from build123d import *

# Parameters (mm, degrees)
SKETCH_R             = 1.375
PAD_DEPTH            = 3
FILLET_R             = 3.5
SKETCH001_W          = 95
SKETCH001_H          = 120
SKETCH001_R          = 1.375
SKETCH001_R_2        = 1.4
SKETCH001_R_3        = 1.403567
PAD001_DEPTH         = 7
SKETCH002_R          = 2.75
POCKET_DEPTH         = 1.75
SKETCH003_W          = 65
SKETCH003_H          = 67.5
POCKET001_DEPTH      = 4
SKETCH004_W          = 65
SKETCH004_H          = 100
PAD002_DEPTH         = 5
SKETCH005_W          = 70
SKETCH005_H          = 102.5
PAD003_DEPTH         = 3
SKETCH006_W          = 70
SKETCH006_H          = 5
POCKET002_DEPTH      = 5
FILLET001_R          = 1.5
SKETCH008_R          = 2.54
SKETCH008_R_2        = 1.27
SKETCH008_R_3        = 9.919017
PAD004_DEPTH         = 2
PAD004_FACE95_R      = 2.54
PAD004_FACE95_R_2    = 1.27
PAD005_DEPTH         = 1
PAD005_FACE94_R      = 2.54
PAD005_FACE94_R_2    = 1.27
PAD006_DEPTH         = 1
SKETCH009_W          = 12.7
SKETCH009_H          = 12.7
POCKET003_DEPTH      = 6
POCKET003_DEPTH_BACK = 1
FILLET002_R          = 1.5
SKETCH010_W          = 12.5
SKETCH010_H          = 10
SKETCH010_W_2        = 70
SKETCH010_H_2        = 7.5
PAD007_DEPTH         = 3
SKETCH015_W          = 45
SKETCH015_H          = 35
POCKET004_DEPTH      = 1
SKETCH028_W          = 1.25
SKETCH028_H          = 105
POCKET005_DEPTH      = 5
SKETCH031_W          = 70
SKETCH031_H          = 5
PAD025_DEPTH         = 15
FILLET007_R          = 4.2
SKETCH033_W          = 70
SKETCH033_H          = 7.5
PAD026_DEPTH         = 3.9
BODY_PLACEMENT_ANGLE = 90


with BuildPart() as part:
    # Sketch → Pad (new body)
    with BuildSketch(Plane.XZ):
        Polygon((6.25, 0), (0, 0), (0, 30), (6.25, 30), (58.75, 30), (65, 30), (65, 0), (58.75, 0), (58.75, 11.25), (6.25, 11.25), align=None)
        with Locations((3.5, 26.5)):
            Circle(SKETCH_R, mode=Mode.SUBTRACT)
        with Locations((61.5, 26.5)):
            Circle(SKETCH_R, mode=Mode.SUBTRACT)
        with Locations((3.5, 3.5)):
            Circle(SKETCH_R, mode=Mode.SUBTRACT)
        with Locations((61.5, 3.5)):
            Circle(SKETCH_R, mode=Mode.SUBTRACT)
    extrude(amount=PAD_DEPTH)

    # Fillet
    fillet_edges = [part.edges().sort_by_distance(p)[0] for p in [
        (0, -1.5, 30),
        (0, -1.5, 0),
        (65, -1.5, 30),
        (65, -1.5, 0),
    ]]
    fillet(fillet_edges, radius=FILLET_R)

    # Sketch001 (on Face5 of Fillet) → Pad001 (join)
    with BuildSketch(Plane.XZ.offset(3)):
        with Locations((32.5, 50)):
            Rectangle(SKETCH001_W, SKETCH001_H)
        with Locations((3.5, 26.5)):
            Circle(SKETCH001_R, mode=Mode.SUBTRACT)
        with Locations((3.5, 3.5)):
            Circle(SKETCH001_R_2, mode=Mode.SUBTRACT)
        with Locations((61.5, 3.5)):
            Circle(SKETCH001_R_2, mode=Mode.SUBTRACT)
        with Locations((61.5, 26.5)):
            Circle(SKETCH001_R_3, mode=Mode.SUBTRACT)
    extrude(amount=PAD001_DEPTH)

    # Sketch002 (on Face29 of Pad001) → Pocket (cut)
    with BuildSketch(Plane.XZ.offset(10)):
        with Locations((3.5, 3.499999)):
            Circle(SKETCH002_R)
        with Locations((3.55131, 26.405157)):
            Circle(SKETCH002_R)
        with Locations((61.5, 26.500002)):
            Circle(SKETCH002_R)
        with Locations((61.561516, 3.466109)):
            Circle(SKETCH002_R)
    extrude(amount=-POCKET_DEPTH, mode=Mode.SUBTRACT)

    # Sketch003 (on Face5 of Pocket) → Pocket001 (cut)
    with BuildSketch(Plane(origin=(0, -3, 0), x_dir=(1, 0, 0), z_dir=(0, 1, 0))):
        with Locations((32.5, -66.25)):
            Rectangle(SKETCH003_W, SKETCH003_H)
    extrude(amount=-POCKET001_DEPTH, mode=Mode.SUBTRACT)

    # Sketch004 (on Face5 of Pocket001) → Pad002 (join)
    with BuildSketch(Plane(origin=(0, -3, 0), x_dir=(1, 0, 0), z_dir=(0, 1, 0))):
        Polygon((0, 5), (65, 5), (70, 5), (70, -100), (80, -100), (80, -110), (-15, -110), (-15, -100), (-5, -100), (-5, 5), align=None)
        with Locations((32.5, -50)):
            Rectangle(SKETCH004_W, SKETCH004_H, mode=Mode.SUBTRACT)
    extrude(amount=PAD002_DEPTH)

    # Sketch005 (on Face22 of Pad002) → Pad003 (join)
    with BuildSketch(Plane(origin=(0, 2, 0), x_dir=(1, 0, 0), z_dir=(0, 1, 0))):
        Polygon((75, 5), (-10, 5), (-10, -100), (-15, -100), (-15, -110), (80, -110), (80, -100), (75, -100), align=None)
        with Locations((32.5, -51.25)):
            Rectangle(SKETCH005_W, SKETCH005_H, mode=Mode.SUBTRACT)
    extrude(amount=PAD003_DEPTH)

    # Sketch006 (on Face34 of Pad003) → Pocket002 (cut)
    with BuildSketch(Plane(origin=(0, 5, 0), x_dir=(1, 0, 0), z_dir=(0, 1, 0))):
        with Locations((32.5, 2.5)):
            Rectangle(SKETCH006_W, SKETCH006_H)
    extrude(amount=-POCKET002_DEPTH, mode=Mode.SUBTRACT)

    # Fillet001
    fillet001_edges = [part.edges().sort_by_distance(p)[0] for p in [
        (32.5, -10, -10),
        (-15, -10, 50),
        (80, -10, 50),
        (32.5, -10, 110),
        (58.811516, -10, 3.466109),
        (58.75, -10, 26.500002),
        (0.80131, -10, 26.405157),
        (0.75, -10, 3.499999),
    ]]
    fillet(fillet001_edges, radius=FILLET001_R)

    # Sketch008 (on Face90 of Fillet001) → Pad004 (join)
    with BuildSketch(Plane(origin=(0, -7, 0), x_dir=(1, 0, 0), z_dir=(0, 1, 0))):
        with Locations((43.18, -96.52)):
            Circle(SKETCH008_R)
        with Locations((43.18, -96.52)):
            Circle(SKETCH008_R_2, mode=Mode.SUBTRACT)
        with Locations((60.96, -96.52)):
            Circle(SKETCH008_R)
        with Locations((60.96, -96.52)):
            Circle(SKETCH008_R_2, mode=Mode.SUBTRACT)
        with Locations((52.07, -81.28)):
            Circle(SKETCH008_R_3)
    extrude(amount=PAD004_DEPTH)

    # Pad004 Face95 → Pad005 (add)
    with BuildSketch(Plane(origin=(43.18, -5, 96.52), x_dir=(1, 0, 0), z_dir=(0, 1, 0))):
        Circle(PAD004_FACE95_R)
        Circle(PAD004_FACE95_R_2, mode=Mode.SUBTRACT)
    extrude(amount=PAD005_DEPTH)

    # Pad005 Face94 → Pad006 (add)
    with BuildSketch(Plane(origin=(60.96, -5, 96.52), x_dir=(1, 0, 0), z_dir=(0, 1, 0))):
        Circle(PAD005_FACE94_R)
        Circle(PAD005_FACE94_R_2, mode=Mode.SUBTRACT)
    extrude(amount=PAD006_DEPTH)

    # Sketch009 (on Face57 of Pad006) → Pocket003 (cut, two sides)
    with BuildSketch(Plane(origin=(0, 2, 0), x_dir=(1, 0, 0), z_dir=(0, 1, 0))) as pocket003_sk:
        with Locations((52.07, -105.41)):
            Rectangle(SKETCH009_W, SKETCH009_H)
    extrude(amount=-POCKET003_DEPTH, mode=Mode.SUBTRACT)
    extrude(pocket003_sk.sketch, amount=POCKET003_DEPTH_BACK, mode=Mode.SUBTRACT)

    # Fillet002
    fillet002_edges = [part.edges().sort_by_distance(p)[0] for p in [
        (45.72, -0.5, 110),
        (52.07, -4, 110),
        (58.42, -0.5, 110),
        (52.07, 3, 110),
    ]]
    fillet(fillet002_edges, radius=FILLET002_R)

    # Sketch010 (on Face29 of Fillet002) → Pad007 (join)
    with BuildSketch(Plane(origin=(0, 5, 0), x_dir=(1, 0, 0), z_dir=(0, 1, 0))):
        with Locations((-8.75, -105)):
            Rectangle(SKETCH010_W, SKETCH010_H)
        with Locations((32.5, -106.25)):
            Rectangle(SKETCH010_W_2, SKETCH010_H_2)
        with Locations((73.75, -105)):
            Rectangle(SKETCH010_W, SKETCH010_H)
    extrude(amount=PAD007_DEPTH)

    # Sketch015 (on Face18 of Pad007) → Pocket004 (cut)
    with BuildSketch(Plane.XZ.offset(10)):
        with Locations((32.5, 15)):
            Rectangle(SKETCH015_W, SKETCH015_H)
    extrude(amount=-POCKET004_DEPTH, mode=Mode.SUBTRACT)

    # Sketch028 (on Face87 of Pocket004) → Pocket005 (cut)
    with BuildSketch(Plane(origin=(0, 5, 0), x_dir=(1, 0, 0), z_dir=(0, 1, 0))):
        with Locations((-9.375, -47.5)):
            Rectangle(SKETCH028_W, SKETCH028_H)
        with Locations((74.375, -47.5)):
            Rectangle(SKETCH028_W, SKETCH028_H)
    extrude(amount=-POCKET005_DEPTH, mode=Mode.SUBTRACT)

    # Sketch031 (on Face16 of Pocket005) → Pad025 (join)
    with BuildSketch(Plane(origin=(0, -3, 0), x_dir=(1, 0, 0), z_dir=(0, 1, 0))):
        with Locations((32.5, 7.5)):
            Rectangle(SKETCH031_W, SKETCH031_H)
    extrude(amount=PAD025_DEPTH)

    # Fillet007
    fillet007_edges = [part.edges().sort_by_distance(p)[0] for p in [
        (-2.5, 12, -7.5),
        (67.5, 12, -7.5),
    ]]
    fillet(fillet007_edges, radius=FILLET007_R)

    # Sketch033 (on Face94 of Fillet007) → Pad026 (join)
    with BuildSketch(Plane(origin=(0, 8, 0), x_dir=(1, 0, 0), z_dir=(0, 1, 0))):
        with Locations((32.5, -106.25)):
            Rectangle(SKETCH033_W, SKETCH033_H)
    extrude(amount=PAD026_DEPTH)


with BuildPart() as part_1:
    # Body placement: moved
    add(part.part.rotate(Axis((0, 0, 0), (1, 0, 0)), BODY_PLACEMENT_ANGLE))


solid = part_1.part
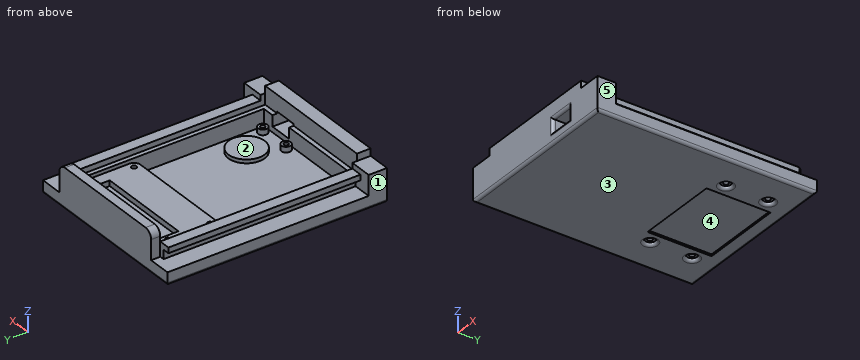
For this review, take the finished solid that the model builds, in its own axes (mm). Face numbers are marked on the shaded views. A direction names the side the tool comes from. Give positions to 0.01 mm unless a question says otherwise; leave off trailing zeros. Loops run counter-clockwise (first coordinate to the right, second up) from the corner with the lowest first, then second, coordinate; pieces in that order, holes last.
Item 1: Insertion check: pin 1 (1.5 mm diameter, centred on x = 43.18, y = -96.52, fed in from +Z); pin 2 (6 mm diameter, centred on y = -3.5, z = 7, fed in from +X); pin 3 (5 mm diameter, centred on x = 72.5, y = -106.5, fed in from +Z). Each pin has a flat end and moves straight along its axis. Give the tip position at first contact, or say it passes through.
Item 2: Take a section at B-B, the plane x = 26.5. State the section outline as (y, z) points, and give its area (3 significant figures).
Item 3: For line 1 along Y through (x, z) = (3.5, -4.5) (3 decimals); line 2 along Y through (x, z) = (61.5, -8.4); line 3 along X through (y, z) = (-3.5, -4.7), list the stretches that pass through material, from the lowest coordinate up.
Item 4: Tool access review of the marked faces 1 and 2: name each direction out of +Z, -Z, +X, -X, +Y, -Y from which nothing blocks a thin tool from reaching the whole face with its end or side.
Item 5: Take a section at A-A, the plane y = -50. State the section outline as (x, z) points, and give its area (3 significant figures).
Item 6: Draft analysis for pull direction X (two halves, no side actions). For the marked faces 3, 4 and 5, state which applies: +X half, -X half, draft (parallel to the pull), parting line (faces both ways), or undercut.
Item 7: Take a section at D-D, the plane y = -80. State the section outline as (x, z) points.
Item 8: Take a section at C-C, the plane z = 10. State the section outline as (x, y) points.
Calculated:
1. pin 1: stops at z = -7
1. pin 2: stops at x = 73.75
1. pin 3: stops at z = 8
2. outline: (-110, -8.5) arc R1.5 ccw to (-108.5, -10) - (-32.5, -10) - (-32.5, -9) - (2.5, -9) - (2.5, -10) - (8.5, -10) arc R1.5 ccw to (10, -8.5) - (10, 12) - (5, 12) - (5, 0) - (0, 0) - (0, -3) - (-11.25, -3) - (-11.25, 0) - (-30, 0) - (-30, -3) - (-32.5, -3) - (-32.5, -7) - (-100, -7) - (-100, 2) - (-102.5, 2) - (-102.5, 11.9) - (-110, 11.9) - close
2. area: 805 mm2
3. line 1: y = -110 to -100, -32.5 to -27.875, -25.125 to -4.9, -2.1 to 10
3. line 2: y = -110 to -29.25, -23.75 to -6.22, -0.72 to 10
3. line 3: x = -15 to 2.1, 4.9 to 60.1, 62.9 to 80
4. face 1: +Z, -Z, -X, +Y, -Y
4. face 2: +Z
5. outline: (-15, -8.5) arc R1.5 ccw to (-13.5, -10) - (78.5, -10) arc R1.5 ccw to (80, -8.5) - (80, -3) - (70, -3) - (70, 2) - (73.75, 2) - (73.75, 5) - (67.5, 5) - (67.5, 2) - (65, 2) - (65, -7) - (0, -7) - (0, 2) - (-2.5, 2) - (-2.5, 5) - (-8.75, 5) - (-8.75, 2) - (-5, 2) - (-5, -3) - (-15, -3) - close
5. area: 492 mm2
6. face 3: draft
6. face 4: undercut
6. face 5: +X half
7. outline: (-15, -8.5) arc R1.5 ccw to (-13.5, -10) - (78.5, -10) arc R1.5 ccw to (80, -8.5) - (80, -3) - (70, -3) - (70, 2) - (73.75, 2) - (73.75, 5) - (67.5, 5) - (67.5, 2) - (65, 2) - (65, -7) - (61.91, -7) - (61.91, -5) - (42.23, -5) - (42.23, -7) - (0, -7) - (0, 2) - (-2.5, 2) - (-2.5, 5) - (-8.75, 5) - (-8.75, 2) - (-5, 2) - (-5, -3) - (-15, -3) - close
8. outline: (-2.5, -110) - (67.5, -110) - (67.5, -102.5) - (-2.5, -102.5) - close; (-1.88, 5) - (66.88, 5) - (66.88, 10) - (-1.88, 10) - close
